For this review, take the finished solid that the model builds, in its own axes (mm). Coordinates: 2 decimals unless noted, no trailing zeros. Order: outer loops, then holes, each group sorted by start corner. A loop starts at its lowest first (then second) coordinate and runs counter-clockwise, first axis right, second up. Notation, with made-up numbers: (34, 32.5) -> (41, 32.5) arc R17 ccw to (41, 40.5) -> close; hole circle Ø8 at (4.5, -8). An arc over 180 degrees is marked (long way). Return JSON: item names as keys, results as strings. Group by question number.
Item 1: Insertion check: pin 1 (1 mm diameter, centred on x = -8, z = 1.5, fed in from -Y). The pin has a flat end and moves straight along its axis. Give the tip position at first contact, or say it passes through.
Item 2: For line 1 along Y through (x, z) = (-7, 0.95); line 2 along X through (y, z) = (9.5, 0.55); line 3 along X through (y, z) = (-6.75, 1.2), list the stretches that pass through material, from the lowest coordinate up.
Item 3: Take a section at B-B (z = 0.65). Write out the cut boundary in (x, y), then the cut area to 3 significant figures.
```python
from build123d import *

# Parameters (mm, degrees)
F0_W     = 47.8917
F0_H     = 22.8092
F1_DEPTH = 2.032
F2_SIZE  = 2.03199


# Not quite as in the source:
# - a fillet or chamfer is up to 0.001 mm smaller than in the source, because OpenCascade refuses the exact size


with BuildPart() as f1:
    # F0 (on Top) → F1 (new body)
    with BuildSketch(Plane.XY):
        Rectangle(F0_W, F0_H)
    extrude(amount=F1_DEPTH)

    # F2 (size 2.032 in the source; OpenCascade refuses exactly that, so slightly less here)
    f2_edges = [f1.edges().sort_by_distance(p)[0] for p in [
        (0, -11.4046, 2.032),
        (-23.94585, 0, 2.032),
        (0, 11.4046, 2.032),
        (23.94585, 0, 2.032),
        (23.94585, -11.4046, 1.016),
        (-23.94585, -11.4046, 1.016),
        (23.94585, 11.4046, 1.016),
        (-23.94585, 11.4046, 1.016),
    ]]
    chamfer(f2_edges, length=F2_SIZE)


solid = f1.part
```
Findings below:
{
 "1": {"pin 1": "stops at y = -10.4"},
 "2": {"line 1": "y = -10.45 to 10.45", "line 2": "x = -23.27 to 23.27", "line 3": "x = -22.75 to 22.75"},
 "3": {"outline": "(-23.3, -9.37) -> (-21.91, -10.75) -> (21.91, -10.75) -> (23.3, -9.37) -> (23.3, 9.37) -> (21.91, 10.75) -> (-21.91, 10.75) -> (-23.3, 9.37) -> close", "area": "998 mm2"}
}
